Job drawing, mm, ordinate dimensions from the low corner. One solid piece. Round coordinates to 2 decimals unless told otherwise and drop trailing zeros. Order: outer loops, then holes, each group sorted by start corner. A loop starts at its lowest first (then second) coordinate and runs counter-clockwise, first axis right, second up. Notation, with made-up numbers: (20.25, 7.5) - (54.25, 7.5) arc R27 cw to (54.25, 38.5) - close; hole circle Ø11 at (52.5, 55). An arc over 180 degrees is marked (long way). Write each question's results on one line, items separated by ' | '. Start each with the question number.
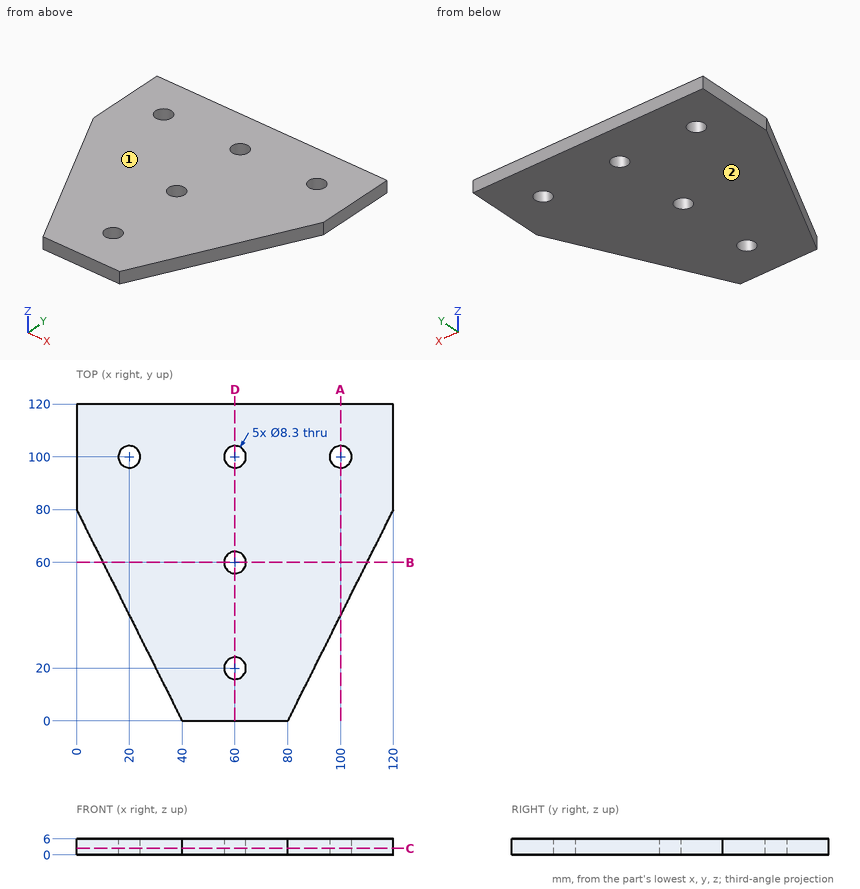
1. Cut at D-D (x = 60). List the corners of the cut face in (y, z).
2. Mould opens along Z. For the marked faces 1 and 2 say: pulls with the +Z half, pulls with the -Z half, needs draft (parallel to the pull), parting line crosses it, or undercut.
3. Wall check: line 1 (X direction, y = 99, z = 0.75); line 2 (X direction, y = 102.5, z = 3.6); line 3 (X direction, y = 56.5, z = 0.4). Give the ranges that are in metal, low to high. Write a range as from..to.
4. Cut at B-B (y = 60). List the corners of the cut face in (x, z).
5. Flat gauge pins, fed straight in: pin 1 Ø2 at (y, z) = (52, 1.5) entering from -X; pin 2 Ø1 at (x, z) = (36.5, 1.5) entering from -Y; pin 3 Ø5 at (x, y) = (100, 100) entering from +Z; pin 4 Ø3 at (x, z) = (105.5, 4.5) entering from -Y. Where does each tip first touch, or does it go through?
6. Cut at C-C (z = 2.45). List the corners of the cut face in (x, y).
7. Cut at A-A (x = 100). List the corners of the cut face in (y, z), plus the area to 3 significant figures.
A:
1) outline: (0, 0) - (15.85, 0) - (15.85, 6) - (0, 6) - close; (24.15, 0) - (55.85, 0) - (55.85, 6) - (24.15, 6) - close; (64.15, 0) - (95.85, 0) - (95.85, 6) - (64.15, 6) - close; (104.15, 0) - (120, 0) - (120, 6) - (104.15, 6) - close
2) face 1: pulls with the +Z half | face 2: pulls with the -Z half
3) line 1: x = 0..15.97, 24.03..55.97, 64.03..95.97, 104.03..120 | line 2: x = 0..16.69, 23.31..56.69, 63.31..96.69, 103.31..120 | line 3: x = 11.75..57.77, 62.23..108.25
4) outline: (10, 0) - (55.85, 0) - (55.85, 6) - (10, 6) - close; (64.15, 0) - (110, 0) - (110, 6) - (64.15, 6) - close
5) pin 1: stops at x = 13.5 | pin 2: stops at y = 6 | pin 3: passes through | pin 4: stops at y = 48
6) outline: (0, 80) - (40, 0) - (80, 0) - (120, 80) - (120, 120) - (0, 120) - close; hole circle Ø8.3 at (20, 100); hole circle Ø8.3 at (60, 20); hole circle Ø8.3 at (60, 60); hole circle Ø8.3 at (60, 100); hole circle Ø8.3 at (100, 100)
7) outline: (40, 0) - (95.85, 0) - (95.85, 6) - (40, 6) - close; (104.15, 0) - (120, 0) - (120, 6) - (104.15, 6) - close | area: 430 mm^2
